Design review of the part built by this model. Coordinates are the model's own, in mm. A direction names the side the tool comes from. Coordinates: 2 decimals unless noted, no trailing zeros. Loops run counter-clockwise (first coordinate to the right, second up) from the corner with the lowest first, then second, coordinate; pieces in that order, holes last. Notation, with made-up numbers: (26, 38.25) -> (58, 38.25) arc R23 cw to (58, 69.25) -> close; hole circle Ø1 at (64.5, 49). An arc over 180 degrees is marked (long way). Use a Markdown table: item, result. Add a question column.
Q1. Take a section at C-C on z = -5. Write out the cut boundary in (x, y), plus the area to 3 significant figures.
Q2. For faces 5 (the face through (123.513, 1.232, -5.195)), 6 (the face through (48, 1.25, -69)), list the 3-axis set-ups (+Z, -Z, +X, -X, +Y, -Y) from which the entire face can be reached by the end or side of a thin tool; tool diameter is ignored.
Q3. For probe 1 along X at (y, z) = (1.9, -5); probe 2 along Z at (x, y) = (5, 1.05); probe 3 along X at (y, z) = (0.6, -13), list the stretches that pass through material, from the lowest coordinate up.
Q4. Clearance check with a flat-ended pin moving along its axis: pin 1 Ø1.8 at (x, z) = (125, -5) entering from +Y. State where the tip first meets the part, or that it passes through.
Q5. Take a section at A-A on x = 64. Write out the cut boundary in (y, z).
Q6. Take a section at D-D on x = 5. Write out the cut boundary in (y, z).
Q7. Take a section at B-B on z = -19. Write out the cut boundary in (x, y).
Q8. Draft analysis for pull direction X (two halves, no side actions). For faces 1 (the face through (3.99, 1.23, -6.11)), 2 (the face through (4.55, 1.23, -73.57)), 3 (the face through (64, 0, -76)), 4 (the face through (0, 1, -39)), state which applies: pulls with the +X half, pulls with the -X half, needs draft (parallel to the pull), parting line crosses it, or undercut.
from build123d import *

# Parameters (mm, degrees)
SKETCH1_W           = 130
SKETCH1_H           = 80
BOSS_EXTRUDE1_DEPTH = 1.25
SKETCH2_W           = 110
SKETCH2_H           = 60
CUT_EXTRUDE1_DEPTH  = 153.648493278
SKETCH3_R           = 1.5
CUT_EXTRUDE2_DEPTH  = 153.648493278
SKETCH6_W           = 130
SKETCH6_H           = 80
SKETCH6_W_2         = 106
SKETCH6_H_2         = 56
BOSS_EXTRUDE2_DEPTH = 1.25
SKETCH7_R           = 1.5
CUT_EXTRUDE4_DEPTH  = 153.648493278


with BuildPart() as part:
    # Sketch1 → Boss-Extrude1 (new body)
    with BuildSketch(Plane(origin=(0, 0, 0), x_dir=(1, 0, 0), z_dir=(0, 1, 0))):
        with Locations((65, 40)):
            Rectangle(SKETCH1_W, SKETCH1_H)
    extrude(amount=BOSS_EXTRUDE1_DEPTH)

    # Sketch2 → Cut-Extrude1 (cut, through all)
    with BuildSketch(Plane.XZ):
        with Locations((65, -40)):
            Rectangle(SKETCH2_W, SKETCH2_H)
    extrude(amount=-CUT_EXTRUDE1_DEPTH, mode=Mode.SUBTRACT)

    # Sketch3 → Cut-Extrude2 (cut, through all)
    with BuildSketch(Plane(origin=(0, 1.25, 0), x_dir=(1, 0, 0), z_dir=(0, 1, 0))):
        with Locations(Location((5, 75, 0), (0, 0, 270))):
            Circle(SKETCH3_R)
        with Locations(Location((125, 75, 0), (0, 0, 270))):
            Circle(SKETCH3_R)
        with Locations(Location((125, 5, 0), (0, 0, 270))):
            Circle(SKETCH3_R)
        with Locations(Location((5, 5, 0), (0, 0, 270))):
            Circle(SKETCH3_R)
    extrude(amount=-CUT_EXTRUDE2_DEPTH, mode=Mode.SUBTRACT)

    # Sketch6 → Boss-Extrude2 (add)
    with BuildSketch(Plane(origin=(0, 1.25, 0), x_dir=(1, 0, 0), z_dir=(0, 1, 0))):
        with Locations((65, 40)):
            Rectangle(SKETCH6_W, SKETCH6_H)
        with Locations((65, 40)):
            Rectangle(SKETCH6_W_2, SKETCH6_H_2, mode=Mode.SUBTRACT)
    extrude(amount=BOSS_EXTRUDE2_DEPTH)

    # Sketch7 → Cut-Extrude4 (cut, through all)
    with BuildSketch(Plane.XZ.offset(-1.25)):
        with Locations(Location((5, -75, 0), (0, 0, 90))):
            Circle(SKETCH7_R)
        with Locations(Location((5, -5, 0), (0, 0, 90))):
            Circle(SKETCH7_R)
        with Locations(Location((125, -5, 0), (0, 0, 90))):
            Circle(SKETCH7_R)
        with Locations(Location((125, -75, 0), (0, 0, 90))):
            Circle(SKETCH7_R)
    extrude(amount=-CUT_EXTRUDE4_DEPTH, mode=Mode.SUBTRACT)


solid = part.part
Answer list:
| question | item | result |
|---|---|---|
| 1 | outline | (0, 0) -> (3.5, 0) -> (3.5, 2.5) -> (0, 2.5) -> close; (6.5, 0) -> (123.5, 0) -> (123.5, 2.5) -> (6.5, 2.5) -> close; (126.5, 0) -> (130, 0) -> (130, 2.5) -> (126.5, 2.5) -> close |
| 1 | area | 310 mm² |
| 2 | face 5 | +Y, -Y |
| 2 | face 6 | -Y |
| 3 | probe 1 | 0 to 3.5, 6.5 to 123.5, 126.5 to 130 |
| 3 | probe 2 | -80 to -76.5, -73.5 to -6.5, -3.5 to 0 |
| 3 | probe 3 | 0 to 10, 120 to 130 |
| 4 | pin 1 | through |
| 5 | outline | (0, -80) -> (2.5, -80) -> (2.5, -68) -> (1.25, -68) -> (1.25, -70) -> (0, -70) -> close; (0, -10) -> (1.25, -10) -> (1.25, -12) -> (2.5, -12) -> (2.5, 0) -> (0, 0) -> close |
| 6 | outline | (0, -80) -> (2.5, -80) -> (2.5, -76.5) -> (0, -76.5) -> close; (0, -73.5) -> (2.5, -73.5) -> (2.5, -6.5) -> (0, -6.5) -> close; (0, -3.5) -> (2.5, -3.5) -> (2.5, 0) -> (0, 0) -> close |
| 7 | outline | (0, 0) -> (10, 0) -> (10, 1.25) -> (12, 1.25) -> (12, 2.5) -> (0, 2.5) -> close; (118, 1.25) -> (120, 1.25) -> (120, 0) -> (130, 0) -> (130, 2.5) -> (118, 2.5) -> close |
| 8 | face 1 | undercut |
| 8 | face 2 | undercut |
| 8 | face 3 | needs draft |
| 8 | face 4 | pulls with the -X half |
